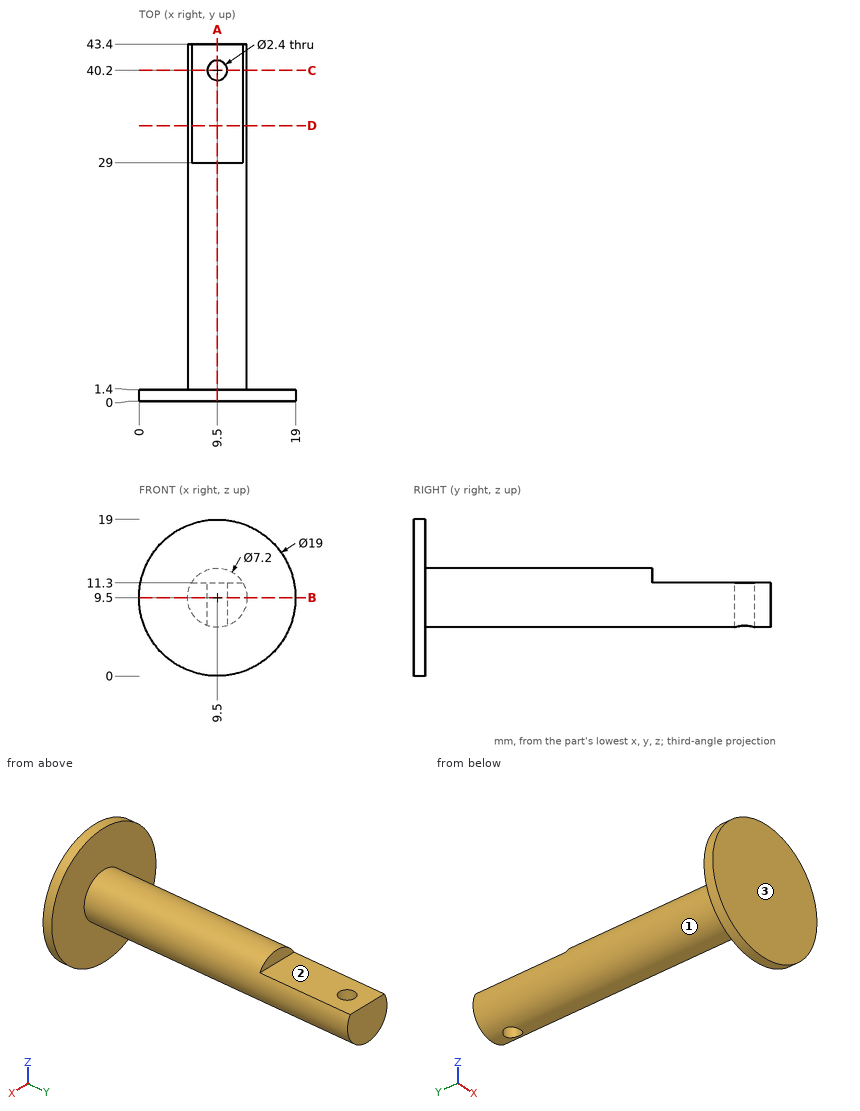
Study the drawing (mm; zero at the part's minimum x, y, z) and answer. A direction names the side the tool comes from. Round coordinates to 2 decimals unless told otherwise and drop trailing zeros. Write each loop counter-clockwise with the first axis right and the second up, starting at its lowest first coordinate (ties: lowest second). Pieces come first, ordered by that corner, then holes. Notation, with made-up numbers: (4, 27.25) -> (38, 27.25) arc R38 cw to (38, 66.25) -> close; hole circle Ø1 at (-11, 27.25). An arc over 180 degrees is marked (long way). Write item = value, one per line.
1) Section A-A on x = 9.5 is taken. Write down the section's boundary in (y, z).
Check values:
outline = (0, 0) -> (1.4, 0) -> (1.4, 5.9) -> (39, 5.9) -> (39, 11.3) -> (29, 11.3) -> (29, 13.1) -> (1.4, 13.1) -> (1.4, 19) -> (0, 19) -> close; (41.4, 5.9) -> (43.4, 5.9) -> (43.4, 11.3) -> (41.4, 11.3) -> close
2) Section D-D on y = 33.5 is taken. Write down the section's boundary in (x, z).
Check values:
outline = (6.38, 11.3) arc R3.6 ccw (long way) to (12.62, 11.3) -> close
3) Section C-C on y = 40.2 is taken. Write down the section's boundary in (x, z), plus the area to 3 significant figures.
Check values:
outline = (6.38, 11.3) arc R3.6 ccw to (8.3, 6.11) -> (8.3, 11.3) -> close; (10.7, 6.11) arc R3.6 ccw to (12.62, 11.3) -> (10.7, 11.3) -> close
area = 20.0 mm²
4) Which of the six approach directions +Z, -Z, +X, -X, +Y, -Y give full straight-line access (tool end or side, diameter ignored) to the marked faces 1, 2 and 3?
Check values:
face_1 = +Y
face_2 = +Z, +X, -X, +Y
face_3 = +Z, -Z, +X, -X, -Y
5) Section B-B on z = 9.5 is taken. Write down the section's boundary in (x, y).
Check values:
outline = (0, 0) -> (19, 0) -> (19, 1.4) -> (13.1, 1.4) -> (13.1, 43.4) -> (5.9, 43.4) -> (5.9, 1.4) -> (0, 1.4) -> close; hole circle Ø2.4 at (9.5, 40.2)
6) Given pin 1 (3 mm diameter, centred on x = 9.5, y = 36.5, fed in from +Z); pin 2 (3 mm diameter, centred on x = 8.5, y = 20, fed in from -Z); pin 3 (1.4 mm diameter, centred on x = 9.5, y = 40.2, fed in from -Z); pin 4 (3 mm diameter, centred on x = 7, y = 20, fed in from -Z), each flat-ended and moving along its own axis, determine where each tip first touches the part or whether it passes through.
Check values:
pin_1 = 11.3
pin_2 = 5.9
pin_3 = through
pin_4 = 6.04
7) Straight lines are drawn through the part: line 1 along Y through (x, z) = (9.5, 7.95); line 2 along X through (y, z) = (40.2, 9.25); line 3 along Y through (x, z) = (4.5, 9.5). For each, find the intervals that lie inside material, in ascending order. Write a range as [from, to].
Check values:
line_1 = [0, 39], [41.4, 43.4]
line_2 = [5.91, 8.3], [10.7, 13.09]
line_3 = [0, 1.4]
